Could you check a few things on this model? Use its own coordinates, in mm. Face numbers are marked on the shaded views. A direction names the side the tool comes from. Round coordinates to 2 decimals unless told otherwise and drop trailing zeros. Write each loop counter-clockwise with the first axis right and the second up, starting at its lowest first coordinate (ties: lowest second). Pieces come first, ordered by that corner, then holes. Notation, with made-up numbers: (39, 48) -> (50, 48) arc R7 cw to (50, 53) -> close; hole circle Ø9 at (5, 52.5). An arc over 180 degrees is marked (long way). One line per question, with ' | ' between items. Start each with the question number.
1. Imagine slicing it at C-C, the plane x = -41.5. List the corners of the cut face in (y, z) for me.
2. For pin 1 Ø8 at (x, z) = (-42, 224.5) entering from -Y; pin 2 Ø12 at (y, z) = (19, -61) entering from +X; pin 3 Ø24 at (x, y) = (20, 152.5) entering from -Z; pin 4 Ø12 at (y, z) = (51.5, -104.5) entering from -X, each with a flat end and sliding along its axis, tell me the tip position at first contact or that it passes through.
3. If I drill on line 1 along X through (y, z) = (118.5, 137.5); line 2 along X through (y, z) = (36, 261.5); line 3 along Z through (x, y) = (-41.5, 118), over which ranges is the centre line in solid material (lowest first)? Write a range as [from, to].
4. Imagine slicing it at B-B, the plane y = 65.5. List the corners of the cut face in (x, z) for me, and give its area (3 significant figures).
5. Imagine slicing it at D-D, the plane z = 224. List the corners of the cut face in (x, y) for me.
6. Imagine slicing it at A-A, the plane y = 39. List the corners of the cut face in (x, z) for me.
7. For the marked faces 1, 2 and 3, which set-ups out of +Z, -Z, +X, -X, +Y, -Y let a thin tool reach every point of the face, with its end or its side?
8. Thinking about a two-plate mould opening in Z: for the marked faces 4, 5 and 6, which applies, released by +Z, released by -Z, zero draft, split by the parting line, or undercut?
Autodesk Inventor part; units mm, degrees
ref_plane "YZ Plane" through (0, 0, 0) normal (1, 0, 0) x (0, 1, 0)
ref_plane "XZ Plane" through (0, 0, 0) normal (0, 1, 0) x (-1, 0, 0)
ref_plane "XY Plane" through (0, 0, 0) normal (0, 0, 1) x (1, 0, 0)
sketch "Sketch3" plane through (0, 0, 0) normal (0, 1, 0) x (-1, 0, 0)
  line L0 (150, 0) -> (-150, 0)
  line L1 (-150, 0) -> (-150, 300)
  line L2 (-150, 300) -> (150, 300)
  line L3 (150, 300) -> (150, 0)
  circle A0 centre (0, 0) radius 150
  arc A1 (0, -150) -> (150, 100) centre (-149.8365, 109.9019) ccw
  arc A2 (-150, 100) -> (0, -150) centre (149.8365, 109.9019) ccw
  dimension "d6" = 300
  dimension "d7" = 300
  dimension "d8" = 100
  dimension "d9" = 100
  dimension "d10" = 300
  dimension "d11" = 300
extrude "Extrusion2" add sketch "Sketch3" along normal blind 100 contours A1 A2 L0 | L0 A2 A0 A1 | A1 A0 A2 L1 L2 L3
sketch "Sketch4" plane through (-150, 0, 300) normal (0, 0, 1) x (1, 0, 0)
  line L0 (75, 0) -> (225, 0)
  line L1 (225, 0) -> (225, 60)
  line L2 (225, 60) -> (75, 60)
  line L3 (75, 60) -> (75, 0)
  line L4 (0, 0) -> (300, 0)
  point P0 (150, 0)
  point P1 (150, 0)
  dimension "d14" = 60
  dimension "d15" = 150
extrude "Extrusion3" cut sketch "Sketch4" against normal through all
sketch "Sketch5" plane through (-75, 60, 300) normal (0, -1, 0) x (1, 0, 0)
  line L0 (0, -388.7146) -> (0, 0)
  line L1 (150, 0) -> (150, -388.7146)
  line L2 (0, -100) -> (150, -100)
  line L3 (150, -100) -> (150, -200)
  line L4 (150, -200) -> (0, -200)
  line L5 (0, -200) -> (0, -100)
  point P0 (75, -300)
  dimension "d18" = 100
  dimension "d19" = 100
extrude "Extrusion4" cut sketch "Sketch5" against normal through all
sketch "Sketch6" plane through (0, 100, 0) normal (0, 1, 0) x (1, 0, 0)
  line L0 (-75, -200) -> (-75, -100)
  line L1 (-75, -100) -> (75, -100)
  line L2 (75, -100) -> (75, -200)
  line L3 (75, -200) -> (-75, -200)
  line L4 (-150, -100) -> (-150, -300)
  line L5 (-150, -300) -> (150, -300)
  line L6 (150, -300) -> (150, -100)
  arc A0 (150, -100) -> (0, 150) centre (-149.8365, -109.9019) ccw
  arc A1 (0, 150) -> (-150, -100) centre (149.8365, -109.9019) ccw
  line L7 (85, -90) -> (-85, -90)
  line L8 (-85, -90) -> (-85, -210)
  line L9 (-85, -210) -> (85, -210)
  line L10 (85, -210) -> (85, -90)
  point P0 (0, 0)
  dimension "d22" = 10
extrude "Extrusion5" add sketch "Sketch6" along normal blind 80 contours L10 L9 L8 L7
sketch "Sketch7" plane through (0, 100, 0) normal (0, 1, 0) x (1, 0, 0)
  line L0 (85, -90) -> (-85, -90) construction
  line L1 (50, -90) -> (-50, -90)
  line L2 (-50, -90) -> (-50, 0)
  line L3 (-50, 0) -> (50, 0)
  line L4 (50, 0) -> (50, -90)
  point P0 (0, 0)
  point P1 (0, -90)
  point P2 (0, 0)
  dimension "d25" = 100
extrude "Extrusion6" add sketch "Sketch7" along normal blind 60
properties part number "GeneralCraftShape3"
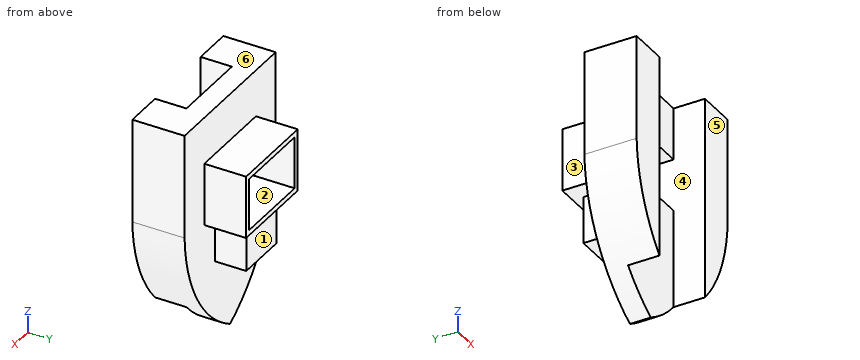
Geometry results:
1) outline: (60, -121.16) -> (100, -121.16) -> (100, 0) -> (160, 0) -> (160, 90) -> (180, 90) -> (180, 100) -> (60, 100) -> close; (60, 200) -> (180, 200) -> (180, 210) -> (100, 210) -> (100, 300) -> (60, 300) -> close
2) pin 1: stops at y = 60 | pin 2: stops at x = 100.78 | pin 3: stops at z = 0 | pin 4: passes through
3) line 1: x = [-85, -75], [75, 85] | line 2: x = [-150, -75], [75, 150] | line 3: z = [0, 100], [200, 210]
4) outline: (-150, 100) arc R300 ccw to (0, -150) arc R300 ccw to (150, 100) -> (150, 300) -> (-150, 300) -> close; hole (-75, 100) -> (75, 100) -> (75, 200) -> (-75, 200) -> close | area: 97,400 mm2
5) outline: (-150, 0) -> (-75, 0) -> (-75, 60) -> (75, 60) -> (75, 0) -> (150, 0) -> (150, 100) -> (-150, 100) -> close
6) outline: (-150, 100) arc R300 ccw to (-75, -88.71) -> (-75, 300) -> (-150, 300) -> close; (75, -88.71) arc R300 ccw to (150, 100) -> (150, 300) -> (75, 300) -> close
7) face 1: -Z, +X, -X, +Y | face 2: +Y, -Y | face 3: +Z, -Z, -X, +Y
8) face 4: undercut | face 5: zero draft | face 6: released by +Z
